Check sheet for the modelled part. Datum: model origin and axes. Units: mm. A direction names the side the tool comes from. Give positions to 0.01 mm unless a question says otherwise; leave off trailing zeros. Order: outer loops, then holes, each group sorted by start corner. A loop starts at its lowest first (then second) coordinate and runs counter-clockwise, first axis right, second up.
```python
from build123d import *

# Parameters (mm, degrees)
CROQUIS1_R              = 9.5
SALIENTE_EXTRUIR1_DEPTH = 7
SALIENTE_EXTRUIR2_DEPTH = 6
CROQUIS3_R              = 4
CORTAR_EXTRUIR1_DEPTH   = 14
CHAFL_N1_SIZE           = 2.5
CHAFL_N1_SIZE2          = 0.531391404


with BuildPart() as part:
    # Croquis1 → Saliente-Extruir1 (new body)
    with BuildSketch(Plane.XY):
        Circle(CROQUIS1_R)
    extrude(amount=SALIENTE_EXTRUIR1_DEPTH)

    # Croquis2 → Saliente-Extruir2 (add)
    with BuildSketch(Plane.XY.offset(7)):
        Polygon((3.711506212, 8.744982655), (-5.717624029, 7.586749994), (-9.429130241, -1.158232661), (-3.711506212, -8.744982655), (5.717624029, -7.586749994), (9.429130241, 1.158232661), align=None)
    extrude(amount=SALIENTE_EXTRUIR2_DEPTH)

    # Croquis3 → Cortar-Extruir1 (cut, through all)
    with BuildSketch(Plane.XY.offset(13)):
        Circle(CROQUIS3_R)
    extrude(amount=-CORTAR_EXTRUIR1_DEPTH, mode=Mode.SUBTRACT)

    # Chaflán1
    chafl_n1_edges = [part.edges().sort_by_distance(p)[0] for p in [
        (6.570318227, 4.951607658, 13),
        (-1.003058908, 8.165866324, 13),
        (-7.573377135, 3.214258666, 13),
        (-6.570318227, -4.951607658, 13),
        (1.003058908, -8.165866324, 13),
        (7.573377135, -3.214258666, 13),
    ]]
    chafl_n1_side = [part.faces().sort_by_distance(p)[0] for p in [
        (-0.97170094, 7.910582237, 13),
    ]]
    chamfer(chafl_n1_edges, length=CHAFL_N1_SIZE, length2=CHAFL_N1_SIZE2, reference=chafl_n1_side[0])


solid = part.part
```
(1) Material ranges on L1, parallel to Y at x = 0, z = 4.75; L2, parallel to X at y = 2.75, z = 11.5; L3, parallel to X at y = 2.25, z = 2.5, recorded low to high.
Response values:
L1: y = -9.5 to -4, 4 to 9.5
L2: x = -7.77 to -2.9, 2.9 to 8.23
L3: x = -9.23 to -3.31, 3.31 to 9.23
(2) Cross-section at C-C on y = 0. Enter the section's corners in (x, z).
Response values:
outline: (-9.5, 0) - (-4, 0) - (-4, 13) - (-6.22, 13) - (-8.94, 12.47) - (-8.94, 7) - (-9.5, 7) - close; (4, 0) - (9.5, 0) - (9.5, 7) - (8.94, 7) - (8.94, 12.47) - (6.22, 13) - (4, 13) - close
(3) Cross-section at A-A on z = 8. Enter the section's corners in (x, y).
Response values:
outline: (-9.43, -1.16) - (-3.71, -8.74) - (5.72, -7.59) - (9.43, 1.16) - (3.71, 8.74) - (-5.72, 7.59) - close; hole circle Ø8 at (0, 0)
(4) Set-up check for faces 5 (the face through (-1, 9, 7)), 6 (the face through (7, 5, 7)), 7 (the face through (0.937, -8.174, 9.696)), 8 (the face through (-6.61, -4.9, 9.7)): record each of +Z, -Z, +X, -X, +Y, -Y from which the full face is reachable in a straight line by a thin tool's end or side.
Response values:
face 5: +Z, -X, +Y
face 6: +Z, +X, +Y
face 7: +Z, +X, -Y
face 8: +Z, -X, -Y
(5) Release check for a two-part mould opening along Y. For faces 1 (the face through (6.61, 4.9, 9.7)), 2 (the face through (-8, 3, 7)), 3 (the face through (-0.867, -3.905, 6.591)), 4 (the face through (-5.63, -4.16, 12.73)) record: released by +Y, released by -Y, zero draft, split by the parting line, or undercut.
Response values:
face 1: released by +Y
face 2: zero draft
face 3: undercut
face 4: released by -Y
(6) Cross-section at B-B on x = -3. Enter the section's corners in (y, z), then the cut area to 3 significant figures.
Response values:
outline: (-9.01, 0) - (-2.65, 0) - (-2.65, 13) - (-5.54, 13) - (-7.07, 12.8) - (-8.66, 12.47) - (-8.66, 7) - (-9.01, 7) - close; (2.65, 0) - (9.01, 0) - (9.01, 7) - (7.92, 7) - (7.92, 12.47) - (5.4, 13) - (2.65, 13) - close
area: 155 mm2
(7) Cross-section at D-D on y = 4.5. Enter the section's corners in (x, z).
Response values:
outline: (-8.37, 0) - (8.37, 0) - (8.37, 7) - (6.91, 7) - (6.91, 12.47) - (3.78, 13) - (-4.31, 13) - (-7.03, 12.47) - (-7.03, 7) - (-8.37, 7) - close
(8) Gauge pin test, flat ends, axial feed: pin 1 Ø3 at (x, y) = (-8, 4) entering from +Z; pin 2 Ø1.5 at (x, y) = (-6.5, 7.5) entering from +Z; pin 3 Ø3 at (x, z) = (-5.5, 2) entering from -Y; pin 4 Ø5 at (x, y) = (0, 0) entering from +Z. Record the tip position at first contact, or that the pin passes through.
Response values:
pin 1: stops at z = 12.64
pin 2: stops at z = 12.48
pin 3: stops at y = -8.62
pin 4: passes through
